from build123d import *

# Parameters (mm, degrees)
SKETCH012_R  = 7
PAD007_DEPTH = 49.5
SKETCH011_R  = 2.5
PAD008_DEPTH = 1.5
CHAMFER_SIZE = 1.2
FILLET002_R  = 1


with BuildPart() as part:
    # Sketch012 → Pad007 (new body)
    with BuildSketch(Plane.XY):
        Circle(SKETCH012_R)
    extrude(amount=PAD007_DEPTH)

    # Sketch011 (on Face3 of Pad007) → Pad008 (join)
    with BuildSketch(Plane.XY.offset(49.5)):
        Circle(SKETCH011_R)
    extrude(amount=PAD008_DEPTH)

    # Chamfer
    chamfer_edges = [part.edges().sort_by_distance(p)[0] for p in [
        (-2.5, 0, 51),
    ]]
    chamfer(chamfer_edges, length=CHAMFER_SIZE)

    # Fillet002
    fillet002_edges = [part.edges().sort_by_distance(p)[0] for p in [
        (-1.3, 0, 51),
    ]]
    fillet(fillet002_edges, radius=FILLET002_R)


solid = part.part
The model under review builds one solid part; all positions refer to its coordinate system, in mm. A direction names the side the tool comes from. Give positions to 0.01 mm unless a question says otherwise; leave off trailing zeros. Order: outer loops, then holes, each group sorted by start corner. A loop starts at its lowest first (then second) coordinate and runs counter-clockwise, first axis right, second up. Notation, with made-up numbers: M 36.5,53 L 95.5,53 A14 cw 95.5,77 Z; hole C 38,65 d11. An arc over 180 degrees is marked long. One line per question, with ' | ' between items. Start each with the question number.
1) Wall thickness on L1, parallel to Z at x = -3.25, y = 2.5; L2, parallel to X at y = -2, z = 40; L3, parallel to X at y = 5.75, z = 21.5: over which ranges is each line inside the solid? List them lowest first. Write a range as from..to.
2) Consider section B-B, the plane y = -3. Give the boundary of the cut face in (x, z).
3) Consider section C-C, the plane z = 3.5. Give the boundary of the cut face in (x, y).
4) For faces 1 (the face through (0, -3, 49.5)), 2 (the face through (6.466, -2.681, 24.404)), list the 3-axis set-ups (+Z, -Z, +X, -X, +Y, -Y) from which the entire face can be reached by the end or side of a thin tool; tool diameter is ignored.
5) Clearance check with flat-ended pins moving along their axes: P1, Ø6, axis at y = 5, z = 10, coming from the -X side; P2, Ø1, axis at y = 4, z = 10.5, coming from the +X side; P3, Ø1, axis at x = 3, z = 38, coming from the +Y side. State where each tip first meets the part, or that it passes through.
6) Consider section A-A, the plane x = 4. Give the boundary of the cut face in (y, z).
Found:
1) L1: z = 0..49.5 | L2: x = -6.71..6.71 | L3: x = -3.99..3.99
2) outline: M -6.32,0 L 6.32,0 L 6.32,49.5 L -6.32,49.5 Z
3) outline: C 0,0 d14
4) face 1: +Z | face 2: +Z, -Z
5) P1: stops at x = -6.71 | P2: stops at x = 6.06 | P3: stops at y = 6.54
6) outline: M -5.74,0 L 5.74,0 L 5.74,49.5 L -5.74,49.5 Z
